Input: part model. Units: mm. Frame: model coordinates. A direction names the side the tool comes from. Coordinates: 2 decimals unless noted, no trailing zeros. Order: outer loops, then holes, each group sorted by start corner. A loop starts at its lowest first (then second) coordinate and runs counter-clockwise, first axis right, second up. Notation, with made-up numbers: (9.25, -14) -> (36.25, -14) arc R12 cw to (36.25, 8) -> close; hole circle Ø1 at (85, 15). An arc over 180 degrees is marked (long way). Use one line per item in the form item = value. Start each with the question number.
1) Access query for faces 4 (the cylindrical face through (1.88, -42.96, 2.99)), 5 (the cylindrical face through (-6.94, -31.24, 1.01)). Directions: +Z, -Z, +X, -X, +Y, -Y. A direction counts if a zero-diameter tool reaches every point of the face in a straight line with its end or side. Return the directions, or none.
2) Ray query, line 1 along Y through (x, z) = (23.5, 0.5); line 2 along X through (y, z) = (-22.5, 2.7); line 3 along X through (y, z) = (2.5, 1.75). Return the intervals inside material, ascending.
3) Pin query (flat end, axial travel): pin 1 (0.6 mm diameter, centred on x = 0, z = 3.5, fed in from +Y); pin 2 (0.5 mm diameter, centred on y = 43.5, z = 3, fed in from +X); pin 3 (25 mm diameter, centred on x = 17, y = -4, fed in from +Z). Return the tip coordinate at first contact, or that it passes through.
4) Section query C-C on x = 37. Output: boundary loops of the cut face in (y, z).
5) Draft query along Y for faces 1 (the flat face through (-10, -31, 2)), 2 (the flat face through (16, 39, 4)), 3 (the flat face through (0, 43.617, 3)). Return one class per face: pulls with the +Y half, pulls with the -Y half, needs draft (parallel to the pull), parting line crosses it, or undercut.
6) Section query A-A on y = 0. Output: boundary loops of the cut face in (x, z).
7) Section query B-B on z = 0.9. Count the separate pieces of the cut face and the enclosed holes in it, then the cut area to 3 significant figures.
8) Section query D-D on y = 16. Output: boundary loops of the cut face in (x, z), then the cut area to 3 significant figures.
from build123d import *

# Parameters (mm, degrees)
SKETCH1_R           = 45
BOSS_EXTRUDE1_DEPTH = 2
SKETCH2_R           = 42
BOSS_EXTRUDE2_DEPTH = 2
SKETCH3_R           = 0.5
SKETCH3_R_2         = 32
CUT_EXTRUDE1_DEPTH  = 64.671029519


with BuildPart() as part:
    # Sketch1 → Boss-Extrude1 (new body)
    with BuildSketch(Plane.XY):
        Circle(SKETCH1_R)
    extrude(amount=BOSS_EXTRUDE1_DEPTH)

    # Sketch2 → Boss-Extrude2 (add)
    with BuildSketch(Plane.XY.offset(2)):
        with BuildLine():
            Line((-1, 43.617499368), (1, 43.617499368))
            Line((1, 43.617499368), (1, 42.98837052))
            ThreePointArc((1, 42.98837052), (0, -43), (-1, 42.98837052))
            Line((-1, 42.98837052), (-1, 43.617499368))
        make_face()
        Circle(SKETCH2_R, mode=Mode.SUBTRACT)
    extrude(amount=BOSS_EXTRUDE2_DEPTH)

    # Sketch3 → Cut-Extrude1 (cut, through all)
    with BuildSketch(Plane.XY.offset(2)):
        with Locations((0, 35)):
            Circle(SKETCH3_R)
        with Locations((8.37604825, 33.98296361)):
            Circle(SKETCH3_R)
        with Locations((16.265311022, 30.990960898)):
            Circle(SKETCH3_R)
        with Locations((23.209293038, 26.197876186)):
            Circle(SKETCH3_R)
        with Locations((28.804435306, 19.882266136)):
            Circle(SKETCH3_R)
        with Locations((32.725568494, 12.411171046)):
            Circle(SKETCH3_R)
        with Locations((34.744810593, 4.218783809)):
            Circle(SKETCH3_R)
        with Locations((34.744810593, -4.218783809)):
            Circle(SKETCH3_R)
        with Locations((32.725568494, -12.411171046)):
            Circle(SKETCH3_R)
        with Locations((28.804435306, -19.882266136)):
            Circle(SKETCH3_R)
        with Locations((23.209293038, -26.197876186)):
            Circle(SKETCH3_R)
        with Locations((16.265311022, -30.990960898)):
            Circle(SKETCH3_R)
        with Locations((8.37604825, -33.98296361)):
            Circle(SKETCH3_R)
        with Locations((0, -35)):
            Circle(SKETCH3_R)
        with Locations((-8.37604825, -33.98296361)):
            Circle(SKETCH3_R)
        with Locations((-16.265311022, -30.990960898)):
            Circle(SKETCH3_R)
        with Locations((-23.209293038, -26.197876186)):
            Circle(SKETCH3_R)
        with Locations((-28.804435306, -19.882266136)):
            Circle(SKETCH3_R)
        with Locations((-32.725568494, -12.411171046)):
            Circle(SKETCH3_R)
        with Locations((-34.744810593, -4.218783809)):
            Circle(SKETCH3_R)
        with Locations((-34.744810593, 4.218783809)):
            Circle(SKETCH3_R)
        with Locations((-32.725568494, 12.411171046)):
            Circle(SKETCH3_R)
        with Locations((-28.804435306, 19.882266136)):
            Circle(SKETCH3_R)
        with Locations((-23.209293038, 26.197876186)):
            Circle(SKETCH3_R)
        with Locations((-16.265311022, 30.990960898)):
            Circle(SKETCH3_R)
        with Locations((-8.37604825, 33.98296361)):
            Circle(SKETCH3_R)
        Circle(SKETCH3_R_2)
    extrude(amount=-CUT_EXTRUDE1_DEPTH, mode=Mode.SUBTRACT)


solid = part.part
Answers below:
q1.face_4 = +Z
q1.face_5 = +Z, -Z
q2.line_1 = -38.38 to -26.6, -25.79 to -21.72, 21.72 to 25.79, 26.6 to 38.38
q2.line_2 = -36.64 to -35.46, 35.46 to 36.64
q2.line_3 = -44.93 to -31.9, 31.9 to 44.93
q3.pin_1 = 43.62
q3.pin_2 = 1
q3.pin_3 = through
q4.outline = (-25.61, 0) -> (25.61, 0) -> (25.61, 2) -> (21.91, 2) -> (21.91, 4) -> (19.87, 4) -> (19.87, 2) -> (-19.87, 2) -> (-19.87, 4) -> (-21.91, 4) -> (-21.91, 2) -> (-25.61, 2) -> close
q5.face_1 = undercut
q5.face_2 = needs draft
q5.face_3 = pulls with the +Y half
q6.outline = (-45, 0) -> (-32, 0) -> (-32, 2) -> (-42, 2) -> (-42, 4) -> (-43, 4) -> (-43, 2) -> (-45, 2) -> close; (32, 0) -> (45, 0) -> (45, 2) -> (43, 2) -> (43, 4) -> (42, 4) -> (42, 2) -> (32, 2) -> close
q7.separate_pieces = 1
q7.enclosed_holes = 27
q7.area = 3,120 mm^2
q8.outline = (-42.06, 0) -> (-27.71, 0) -> (-27.71, 2) -> (-38.83, 2) -> (-38.83, 4) -> (-39.91, 4) -> (-39.91, 2) -> (-42.06, 2) -> close; (27.71, 0) -> (42.06, 0) -> (42.06, 2) -> (39.91, 2) -> (39.91, 4) -> (38.83, 4) -> (38.83, 2) -> (27.71, 2) -> close
q8.area = 61.7 mm^2
